Can you work these out from the model? Positions are in its coordinate system, mm. A direction names the side the tool comes from. Coordinates: 2 decimals unless noted, no trailing zeros. Order: outer loops, then holes, each group sorted by start corner. A loop starts at its lowest first (then second) coordinate and runs counter-clockwise, first axis right, second up. Notation, with made-up numbers: (29.5, 46.5) -> (49.5, 46.5) arc R18 cw to (49.5, 69.5) -> close; hole circle Ø1 at (73.25, 36). An arc over 180 degrees is marked (long way). Use a Markdown table: item, result. Add a question column.
1. For faces 1 (the flat face through (-199, -50, -182)), 2 (the flat face through (-197, -78.922, -463)), 3 (the cylindrical face through (-197.2, -27.15, -84.89)), which set-ups out of +Z, -Z, +X, -X, +Y, -Y let a thin tool reach every point of the face, with its end or its side?
2. Suppose I cut it at B-B, the plane y = 0. List the corners of the cut face in (x, z) for me, then the cut area to 3 significant figures.
3. If I drill on line 1 along X through (y, z) = (-20.5, -30); line 2 along Y through (x, z) = (1.75, 0); line 3 along Y through (x, z) = (-335, -434), over which ranges is the centre line in solid material (lowest first)? Write a range as from..to.
4. We'd pull the mould along Y, two halves only. Please class faces 4 (the cylindrical face through (-401.479, -19.524, -4.336)), 5 (the flat face through (-197, -79.922, -450)), 6 (the flat face through (-400, -14, -297)), 7 (the cylindrical face through (-197.2, -73.98, -267.31)): pulls with the +Y half, pulls with the -Y half, needs draft (parallel to the pull), parting line crosses it, or undercut.
5. Suppose I cut it at C-C, the plane z = -320.5. List the corners of the cut face in (x, y) for me, then the cut area to 3 significant figures.
6. For pin 1 Ø5 at (x, y) = (-303.5, -26) entering from -Z; pin 2 Ø24 at (y, z) = (0, 0) entering from +X; pin 3 Ø5 at (x, y) = (-288.5, -13.5) entering from -Z; pin 4 Ø1 at (x, y) = (-293.5, 29) entering from +Z, each with a flat end and sliding along its axis, tell me the tip position at first contact or that it passes through.
7. Suppose I cut it at D-D, the plane y = -36. List the corners of the cut face in (x, z) for me.
8. Suppose I cut it at A-A, the plane x = -275.5. List the corners of the cut face in (y, z) for me, then the cut area to 3 significant figures.
```python
from build123d import *

# Parameters (mm, degrees)
SKETCH_1_R      = 50
SKETCH_1_R_2    = 20
EXTRUDE_1_DEPTH = 3
EXTRUDE_2_DEPTH = 400
SKETCH_3_R      = 20
EXTRUDE_3_DEPTH = 3


with BuildPart() as part:
    # 草图1 → 凸台-拉伸1 (new body)
    with BuildSketch(Plane(origin=(0, 0, 0), x_dir=(0, 0, -1), z_dir=(1, 0, 0))):
        with BuildLine():
            ThreePointArc((50, 0), (35.355339059, -35.355339059), (0, -50))
            Line((0, -50), (192.417140489, -50))
            ThreePointArc((192.417140489, -50), (211.551312107, -53.806023374), (227.772479548, -64.644660941))
            Line((227.772479548, -64.644660941), (228.405158627, -65.277340019))
            ThreePointArc((228.405158627, -65.277340019), (244.626326068, -76.115977585), (263.760497686, -79.92200096))
            Line((263.760497686, -79.92200096), (631.54077851, -79.92200096))
            ThreePointArc((631.54077851, -79.92200096), (634.479494864, -77.525280493), (632.72269013, -74.164631757))
            Line((632.72269013, -74.164631757), (352.484009, 45.956153386))
            ThreePointArc((352.484009, 45.956153386), (342.840140888, 48.978605887), (332.785482, 50))
            Line((332.785482, 50), (0, 50))
            ThreePointArc((0, 50), (35.355339059, 35.355339059), (50, 0))
        make_face()
        Circle(SKETCH_1_R)
        Circle(SKETCH_1_R_2, mode=Mode.SUBTRACT)
    extrude(amount=EXTRUDE_1_DEPTH)

    # 草图2 → 凸台-拉伸2 (add)
    with BuildSketch(Plane.ZY):
        with BuildLine():
            ThreePointArc((-233.606386859, -60.015816693), (-267.811656592, -74.11426689), (-304.494792617, -78.92200096))
            Line((-304.494792617, -78.92200096), (-625.869496691, -78.92200096))
            Line((-625.869496691, -78.92200096), (-631.54077851, -79.92200096))
            Line((-631.54077851, -79.92200096), (-263.760497686, -79.92200096))
            ThreePointArc((-263.760497686, -79.92200096), (-244.626326068, -76.115977585), (-228.405158627, -65.277340019))
            Line((-228.405158627, -65.277340019), (-227.772479548, -64.644660941))
            ThreePointArc((-227.772479548, -64.644660941), (-211.551312107, -53.806023374), (-192.417140489, -50))
            Line((-192.417140489, -50), (-170.764869856, -50))
            ThreePointArc((-170.764869856, -50), (-83.751443835, -26.590589439), (-12.213025887, 28.19619335))
            ThreePointArc((-12.213025887, 28.19619335), (-12.840107981, 28.661683678), (-13.582379077, 28.418894018))
            ThreePointArc((-13.582379077, 28.418894018), (-93.185539951, -28.785672237), (-189.104289812, -49))
            Line((-189.104289812, -49), (-192.417140489, -49))
            ThreePointArc((-192.417140489, -49), (-213.907702397, -51.157903364), (-233.606386859, -60.015816693))
        make_face()
    extrude(amount=EXTRUDE_2_DEPTH)

    # 草图3 → 凸台-拉伸3 (add)
    with BuildSketch(Plane.ZY.offset(400)):
        with BuildLine():
            Line((-352.484009, 45.956153386), (-632.72269013, -74.164631757))
            ThreePointArc((-632.72269013, -74.164631757), (-634.479494864, -77.525280493), (-631.54077851, -79.92200096))
            Line((-631.54077851, -79.92200096), (-625.869496691, -78.92200096))
            Line((-625.869496691, -78.92200096), (-304.494792617, -78.92200096))
            ThreePointArc((-304.494792617, -78.92200096), (-267.811656592, -74.11426689), (-233.606386859, -60.015816693))
            ThreePointArc((-233.606386859, -60.015816693), (-213.907702397, -51.157903364), (-192.417140489, -49))
            Line((-192.417140489, -49), (-189.104289812, -49))
            ThreePointArc((-189.104289812, -49), (-93.185539951, -28.785672237), (-13.582379077, 28.418894018))
            ThreePointArc((-13.582379077, 28.418894018), (-12.840107981, 28.661683678), (-12.213025887, 28.19619335))
            ThreePointArc((-12.213025887, 28.19619335), (-83.751443835, -26.590589439), (-170.764869856, -50))
            Line((-170.764869856, -50), (0, -50))
            ThreePointArc((0, -50), (50, 0), (0, 50))
            Line((0, 50), (-332.785482, 50))
            ThreePointArc((-332.785482, 50), (-342.840140888, 48.978605887), (-352.484009, 45.956153386))
        make_face()
        Circle(SKETCH_3_R, mode=Mode.SUBTRACT)
        with BuildLine():
            ThreePointArc((-170.764869856, -50), (-83.751443835, -26.590589439), (-12.213025887, 28.19619335))
            ThreePointArc((-12.213025887, 28.19619335), (-12.840107981, 28.661683678), (-13.582379077, 28.418894018))
            ThreePointArc((-13.582379077, 28.418894018), (-93.185539951, -28.785672237), (-189.104289812, -49))
            Line((-189.104289812, -49), (-192.417140489, -49))
            ThreePointArc((-192.417140489, -49), (-213.907702397, -51.157903364), (-233.606386859, -60.015816693))
            ThreePointArc((-233.606386859, -60.015816693), (-267.811656592, -74.11426689), (-304.494792617, -78.92200096))
            Line((-304.494792617, -78.92200096), (-625.869496691, -78.92200096))
            Line((-625.869496691, -78.92200096), (-631.54077851, -79.92200096))
            Line((-631.54077851, -79.92200096), (-263.760497686, -79.92200096))
            ThreePointArc((-263.760497686, -79.92200096), (-244.626326068, -76.115977585), (-228.405158627, -65.277340019))
            Line((-228.405158627, -65.277340019), (-227.772479548, -64.644660941))
            ThreePointArc((-227.772479548, -64.644660941), (-211.551312107, -53.806023374), (-192.417140489, -50))
            Line((-192.417140489, -50), (-170.764869856, -50))
        make_face()
    extrude(amount=EXTRUDE_3_DEPTH)


solid = part.part
```
Worked out:
| question | item | result |
|---|---|---|
| 1 | face 1 | +Z, +X, -X, -Y |
| 1 | face 2 | -Z, +Y |
| 1 | face 3 | +Z, -Y |
| 2 | outline | (-403, -459.7) -> (-400, -459.7) -> (-400, -44.57) -> (0, -44.57) -> (0, -459.7) -> (3, -459.7) -> (3, -20) -> (0, -20) -> (0, -41.84) -> (-400, -41.84) -> (-400, -20) -> (-403, -20) -> close; (-403, 20) -> (-400, 20) -> (-400, 50) -> (-403, 50) -> close; (0, 20) -> (3, 20) -> (3, 50) -> (0, 50) -> close |
| 2 | area | 3,910 mm² |
| 3 | line 1 | x = -403..-400, 0..3 |
| 3 | line 2 | y = -50..-20, 20..50 |
| 3 | line 3 | y = -79.92..-78.92 |
| 4 | face 4 | undercut |
| 4 | face 5 | pulls with the -Y half |
| 4 | face 6 | needs draft |
| 4 | face 7 | pulls with the +Y half |
| 5 | outline | (-403, -79.92) -> (3, -79.92) -> (3, 50) -> (0, 50) -> (0, -78.92) -> (-400, -78.92) -> (-400, 50) -> (-403, 50) -> close |
| 5 | area | 1,180 mm² |
| 6 | pin 1 | stops at z = -92.54 |
| 6 | pin 2 | passes through |
| 6 | pin 3 | stops at z = -68.28 |
| 6 | pin 4 | stops at z = -12.46 |
| 7 | outline | (-403, -543.69) -> (-400, -543.69) -> (-400, -111.58) -> (0, -111.58) -> (0, -543.69) -> (3, -543.69) -> (3, 34.7) -> (0, 34.7) -> (0, -105.58) -> (-400, -105.58) -> (-400, 34.7) -> (-403, 34.7) -> close |
| 8 | outline | (-79.92, -631.54) -> (-78.92, -625.87) -> (-78.92, -304.49) arc R142.35 cw to (-60.02, -233.61) arc R67.26 ccw to (-49, -192.42) -> (-49, -189.1) arc R237.68 cw to (28.42, -13.58) arc R0.85 ccw to (28.2, -12.21) arc R232.07 ccw to (-50, -170.76) -> (-50, -192.42) arc R50 cw to (-64.64, -227.77) -> (-65.28, -228.41) arc R50 ccw to (-79.92, -263.76) -> close |
| 8 | area | 1,260 mm² |
